```python
from build123d import *

# Parameters (mm, degrees)
SKETCH1_W                                        = 75
SKETCH1_H                                        = 22
BOSS_EXTRUDE1_DEPTH                              = 22
CBORE_FOR_M10_SOCKET_HEAD_CAP_SCREW1_D           = 12
CBORE_FOR_M10_SOCKET_HEAD_CAP_SCREW1_CBORE_D     = 18
CBORE_FOR_M10_SOCKET_HEAD_CAP_SCREW1_CBORE_DEPTH = 11.366
CHAMFER1_SIZE                                    = 5


with BuildPart() as part:
    # Sketch1 → Boss-Extrude1 (new body)
    with BuildSketch(Plane(origin=(0, 0, 0), x_dir=(1, 0, 0), z_dir=(0, 1, 0))):
        with Locations((0, 11)):
            Rectangle(SKETCH1_W, SKETCH1_H)
    extrude(amount=BOSS_EXTRUDE1_DEPTH)

    # CBORE for M10 Socket Head Cap Screw1 (through all)
    with Locations(Plane.XY):
        with Locations((25, 11), (-25, 11)):
            CounterBoreHole(CBORE_FOR_M10_SOCKET_HEAD_CAP_SCREW1_D / 2, CBORE_FOR_M10_SOCKET_HEAD_CAP_SCREW1_CBORE_D / 2, CBORE_FOR_M10_SOCKET_HEAD_CAP_SCREW1_CBORE_DEPTH)

    # Chamfer1
    # the kernel refuses this chamfer: 5 mm, written as the material it takes off along each edge
    with BuildSketch(Plane(origin=(37.5, -12.85841494, 0), x_dir=(-0.9996219169112968, 0, 0.027495876610586372), z_dir=(0, 1, 0))) as chamfer1_piece_1:
        Polygon((CHAMFER1_SIZE * 0.999621916911, -CHAMFER1_SIZE * 0.0274958766106), (-CHAMFER1_SIZE * 0.0274958766106, -CHAMFER1_SIZE * 0.999621916911), (0, 0), align=None)
    extrude(amount=47.71682988, mode=Mode.SUBTRACT)
    with BuildSketch(Plane(origin=(-37.5, -12.85841494, 0), x_dir=(0.9996219169112968, 0, 0.027495876610586372), z_dir=(0, 1, 0))) as chamfer1_piece_2:
        Polygon((CHAMFER1_SIZE * 0.999621916911, CHAMFER1_SIZE * 0.0274958766106), (-CHAMFER1_SIZE * 0.0274958766106, CHAMFER1_SIZE * 0.999621916911), (0, 0), align=None)
    extrude(amount=47.71682988, mode=Mode.SUBTRACT)


solid = part.part
```
Verification items for the finished model (mm, model axes). A direction names the side the tool comes from. Round coordinates to 2 decimals unless told otherwise and drop trailing zeros. Write each loop counter-clockwise with the first axis right and the second up, starting at its lowest first coordinate (ties: lowest second). Pieces come first, ordered by that corner, then holes.
1. Draft check along X on faces 1 (the flat face through (-35, 10.8, -2.5)), 2 (the flat face through (0, 11, 0)), 3 (the flat face through (31, 9, -11.366)), 4 (the flat face through (35, 10.8, -2.5)). Enter one of: +X half, -X half, draft (parallel to the pull), parting line (faces both ways), or undercut.
2. Section check A-A on x = 25. Enter the section's corners in (y, z), plus the area to 3 significant figures.
3. Section check B-B on y = 11. Enter the section's corners in (x, z), plus the area to 3 significant figures.
4. Scan lines: L1, parallel to X at y = 11, z = -7.75; L2, parallel to Y at x = 25, z = -2.5; L3, parallel to Y at x = 25, z = -19.5. Record each from-to range of solid material in increasing order.
5. Gauge pin test, flat end, axial feed: P1, Ø9, axis at x = 23, y = 14, coming from the +Z side. Record the tip position at first contact, or that the pin passes through.
6. Section check C-C on z = -6.75. Enter the section's corners in (x, y), plus the area to 3 significant figures.
7. Access from +Z, -Z, +X, -X, +Y, -Y to the whole of each face (thin tool, end or side, straight path). Record for faces 5 (the flat face through (-1, 22, -11)), 6 (the flat face through (-19, 9, -11.366)).
8. Section check D-D on x = -18. Enter the section's corners in (y, z).
Answer:
1. face 1: -X half
1. face 2: draft
1. face 3: undercut
1. face 4: +X half
2. outline: (0, -22) - (5, -22) - (5, -11.37) - (2, -11.37) - (2, 0) - (0, 0) - close; (17, -22) - (22, -22) - (22, 0) - (20, 0) - (20, -11.37) - (17, -11.37) - close
2. area: 152 mm2
3. outline: (-37.5, -22) - (-31, -22) - (-31, -11.37) - (-34, -11.37) - (-34, -1.5) - (-37.5, -5) - close; (-19, -22) - (19, -22) - (19, -11.37) - (16, -11.37) - (16, 0) - (-16, 0) - (-16, -11.37) - (-19, -11.37) - close; (31, -22) - (37.5, -22) - (37.5, -5) - (34, -1.5) - (34, -11.37) - (31, -11.37) - close
3. area: 963 mm2
4. L1: x = -37.5 to -34, -16 to 16, 34 to 37.5
4. L2: y = 0 to 2, 20 to 22
4. L3: y = 0 to 5, 17 to 22
5. P1: stops at z = -11.37
6. outline: (-37.5, 0) - (37.5, 0) - (37.5, 22) - (-37.5, 22) - close; hole circle Ø18 at (-25, 11); hole circle Ø18 at (25, 11)
6. area: 1,140 mm2
7. face 5: +Z, -Z, +X, -X, +Y
7. face 6: +Z
8. outline: (0, -22) - (22, -22) - (22, 0) - (16.66, 0) - (16.66, -11.37) - (5.34, -11.37) - (5.34, 0) - (0, 0) - close
